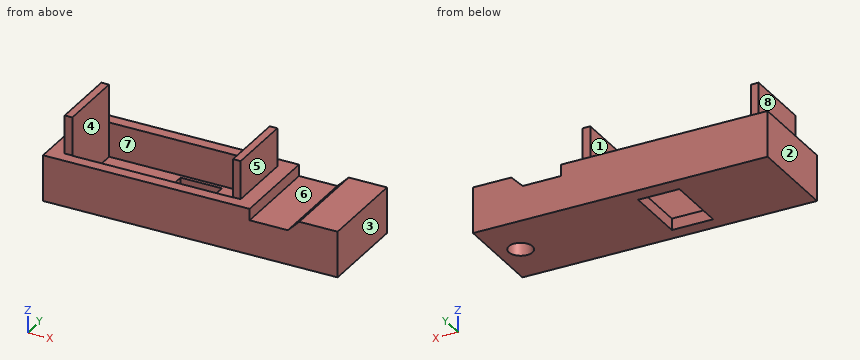
from build123d import *

# Parameters (mm, degrees)
SKETCH_1_W          = 27
SKETCH_1_H          = 12
SKETCH_1_W_2        = 21
SKETCH_1_H_2        = 9
EXTRUDE_1_DEPTH     = 6
SKETCH_2_W          = 21
SKETCH_2_H          = 9
EXTRUDE_2_DEPTH     = 1.5
SKETCH_3_W          = 5.4
SKETCH_3_H          = 8.2
CUT_EXTRUDE_1_DEPTH = 2.5
SKETCH_4_W          = 1
SKETCH_4_H          = 8.9
EXTRUDE_3_DEPTH     = 5
EXTRUDE_5_DEPTH     = 12
SKETCH_9_R          = 1.55
CUT_EXTRUDE_2_DEPTH = 3.5


with BuildPart() as part:
    # 草图1 → 凸台-拉伸1 (new body)
    with BuildSketch(Plane.XY):
        Rectangle(SKETCH_1_W, SKETCH_1_H)
        Rectangle(SKETCH_1_W_2, SKETCH_1_H_2, mode=Mode.SUBTRACT)
    extrude(amount=EXTRUDE_1_DEPTH)

    # 草图2 → 凸台-拉伸2 (add)
    with BuildSketch(Plane(origin=(0, 0, 0), x_dir=(-1, 0, 0), z_dir=(0, 0, -1))):
        Rectangle(SKETCH_2_W, SKETCH_2_H)
    extrude(amount=-EXTRUDE_2_DEPTH)

    # 草图3 → 切除-拉伸1 (cut, through all)
    with BuildSketch(Plane.XY.offset(1.5)):
        with Locations((1.8, -0.1)):
            Rectangle(SKETCH_3_W, SKETCH_3_H)
    extrude(amount=-CUT_EXTRUDE_1_DEPTH, mode=Mode.SUBTRACT)

    # 草图4 → 凸台-拉伸3 (add)
    with BuildSketch(Plane.XY.offset(6)):
        with Locations((-11, 0)):
            Rectangle(SKETCH_4_W, SKETCH_4_H)
        with Locations((11, 0)):
            Rectangle(SKETCH_4_W, SKETCH_4_H)
    extrude(amount=EXTRUDE_3_DEPTH)

    # 草图8 → 凸台-拉伸5 (add)
    with BuildSketch(Plane(origin=(0, 6, 0), x_dir=(1, 0, 0), z_dir=(0, 1, 0))):
        Polygon((13.5, -4.5), (18.5, -4.5), (20, -6), (25, -6), (25, 0), (20, 0), (13.5, 0), (13.5, -1.5), align=None)
    extrude(amount=-EXTRUDE_5_DEPTH)

    # 草图9 → 切除-拉伸2 (cut)
    with BuildSketch(Plane(origin=(0, 0, 0), x_dir=(-1, 0, 0), z_dir=(0, 0, -1))):
        with Locations((-22, 0)):
            Circle(SKETCH_9_R)
    extrude(amount=-CUT_EXTRUDE_2_DEPTH, mode=Mode.SUBTRACT)


solid = part.part
The listing builds one solid part. Answer for the finished solid, in the listing's coordinates (mm). Face numbers are marked on the shaded views. A direction names the side the tool comes from. Round coordinates to 2 decimals unless told otherwise and drop trailing zeros. Order: outer loops, then holes, each group sorted by start corner. A loop starts at its lowest first (then second) coordinate and runs counter-clockwise, first axis right, second up. Notation, with made-up numbers: (72.5, -16.75) - (105.5, -16.75) arc R24 cw to (105.5, 3.25) - close; hole circle Ø8 at (70, -19.5). An arc over 180 degrees is marked (long way). Write item = value, one per line. Start each with the question number.
1) Section A-A, the plane z = 7.5 is taken. Write down the section's boundary in (x, y).
2) Given pin 1 (3.5 mm diameter, centred on x = 5, y = 1, fed in from +Z); pin 2 (4 mm diameter, centred on x = 21.5, y = 2, fed in from +Z); pin 3 (4 mm diameter, centred on y = 0, z = 9, fed in from -X); pin 4 (3.5 mm diameter, centred on x = 22.5, y = -0.5, fed in from -Z), each flat-ended and moving along its own axis, determine where each tip first touches the part or whether it passes through.
3) For the marked faces 5, 6, 7 and 8, determine the directions among +Z, -Z, +X, -X, +Y, -Y from which every point of the face is accessible in a straight line to the end or side of a thin tool.
4) Straight lines are drawn through the part: L1, parallel to X at y = -4, z = 2.75; L2, parallel to X at y = -1.25, z = 5; L3, parallel to Y at x = 22, z = 2.35. For each, find the intervals that lie inside material, in ascending order.
5) Section C-C, the plane y = 0 is taken. Write down the section's boundary in (x, z).
6) For a pull along X with two mould halves and no side action, classify the marked faces 1, 2, 3 and 4 as released by +X, released by -X, zero draft, split by the parting line, or undercut.
7) Section B-B, the plane x = 4 is taken. Write down the section's boundary in (y, z).
8) Section D-D, the plane z = 5.25 is taken. Write down the section's boundary in (x, y).
Results list:
q1.outline = (-11.5, -4.45) - (-10.5, -4.45) - (-10.5, 4.45) - (-11.5, 4.45) - close; (10.5, -4.45) - (11.5, -4.45) - (11.5, 4.45) - (10.5, 4.45) - close
q2.pin_1 = 1.5
q2.pin_2 = 6
q2.pin_3 = -11.5
q2.pin_4 = 0
q3.face_5 = +Z, +X, +Y, -Y
q3.face_6 = +Z, +Y, -Y
q3.face_7 = +Z
q3.face_8 = +Z, -X, +Y, -Y
q4.L1 = -13.5 to -10.5, 10.5 to 25
q4.L2 = -13.5 to -10.5, 10.5 to 13.5, 19 to 25
q4.L3 = -6 to -1.55, 1.55 to 6
q5.outline = (-13.5, 0) - (-0.9, 0) - (-0.9, 1.5) - (-10.5, 1.5) - (-10.5, 11) - (-11.5, 11) - (-11.5, 6) - (-13.5, 6) - close; (4.5, 0) - (20.45, 0) - (20.45, 3.5) - (23.55, 3.5) - (23.55, 0) - (25, 0) - (25, 6) - (20, 6) - (18.5, 4.5) - (13.5, 4.5) - (13.5, 6) - (11.5, 6) - (11.5, 11) - (10.5, 11) - (10.5, 1.5) - (4.5, 1.5) - close
q6.face_1 = undercut
q6.face_2 = released by -X
q6.face_3 = released by +X
q6.face_4 = undercut
q7.outline = (-6, 0) - (-4.2, 0) - (-4.2, 1.5) - (-4.5, 1.5) - (-4.5, 6) - (-6, 6) - close; (4, 0) - (6, 0) - (6, 6) - (4.5, 6) - (4.5, 1.5) - (4, 1.5) - close
q8.outline = (-13.5, -6) - (13.5, -6) - (13.5, 6) - (-13.5, 6) - close; (19.25, -6) - (25, -6) - (25, 6) - (19.25, 6) - close; hole (-10.5, -4.5) - (10.5, -4.5) - (10.5, 4.5) - (-10.5, 4.5) - close
